Check sheet for the drawn part. Datum: minimum x, y, z corner. Units: mm. A direction names the side the tool comes from. Coordinates: 2 decimals unless noted, no trailing zeros. Write each loop counter-clockwise with the first axis right and the second up, starting at its lowest first coordinate (ties: lowest second). Pieces come first, ordered by that corner, then holes. Notation, with made-up numbers: M 78,45 L 119,45 A19 ccw 119,52 Z; hole C 34,-11.5 d4. An arc over 180 degrees is marked long. Answer in a Markdown table with one row per item.
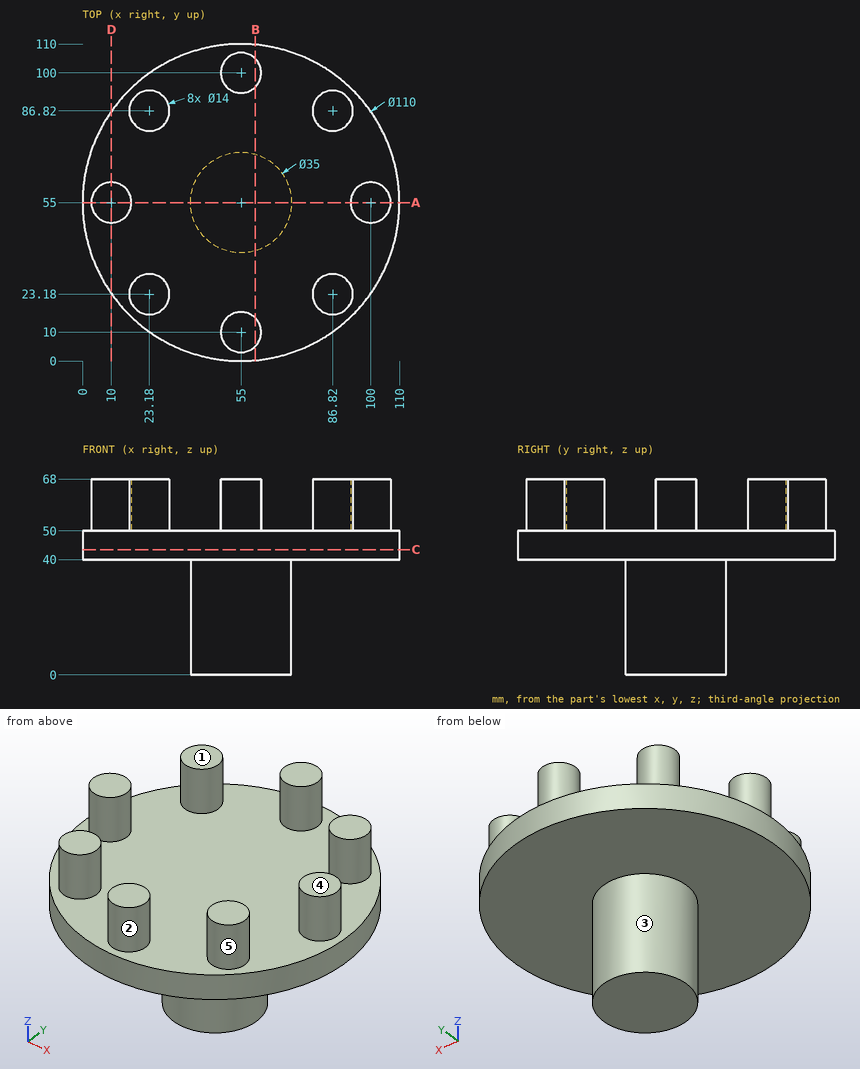
1) Sectioned sample at C-C (z = 43.5). Record the cut outline in (x, y), then the cut area to 3 significant figures.
Response values:
| item | result |
|---|---|
| outline | C 55,55 d110 |
| area | 9,500 mm² |
2) Tool access check on the marked faces 1 and 2. Record the directions out of +Z, -Z, +X, -X, +Y, -Y that give a thin tool (end or side, any length) a straight path to the whole face; none if there is none.
Response values:
| item | result |
|---|---|
| face 1 | +Z, +X, -X, +Y, -Y |
| face 2 | +Z |
3) Thickness scan on L1, parallel to Z at x = 104.5, y = 59.5; L2, parallel to Z at x = 94, y = 37; L3, parallel to Y at x = 50.5, z = 54. Record the ranges inside material, lowest first. Write a range as [from, to].
Response values:
| item | result |
|---|---|
| L1 | z = [40, 68] |
| L2 | z = [40, 50] |
| L3 | y = [4.64, 15.36], [94.64, 105.36] |
4) Sectioned sample at A-A (y = 55). Record the cut outline in (x, z).
Response values:
| item | result |
|---|---|
| outline | M 0,40 L 37.5,40 L 37.5,0 L 72.5,0 L 72.5,40 L 110,40 L 110,50 L 107,50 L 107,68 L 93,68 L 93,50 L 17,50 L 17,68 L 3,68 L 3,50 L 0,50 Z |
5) Depth check by flat-ended pin: pin 1 (10 mm diameter, centred on x = 31.5, y = 41.5, fed in from -Z); pin 2 (3 mm diameter, centred on y = 41, z = 28.5, fed in from -X); pin 3 (12 mm diameter, centred on x = 17, y = 68, fed in from +Z). Enter the tip coordinate at first touch or a pass-through.
Response values:
| item | result |
|---|---|
| pin 1 | stops at z = 40 |
| pin 2 | stops at x = 42.75 |
| pin 3 | stops at z = 50 |
6) Sectioned sample at B-B (x = 60). Record the cut outline in (y, z), then the cut area to 3 significant figures.
Response values:
| item | result |
|---|---|
| outline | M 0.23,40 L 38.23,40 L 38.23,0 L 71.77,0 L 71.77,40 L 109.77,40 L 109.77,50 L 104.9,50 L 104.9,68 L 95.1,68 L 95.1,50 L 14.9,50 L 14.9,68 L 5.1,68 L 5.1,50 L 0.23,50 Z |
| area | 2,790 mm² |
7) Release check for a two-part mould opening along X. For the marked faces 3, 4 and 5 record: +X half, -X half, draft (parallel to the pull), parting line (faces both ways), or undercut.
Response values:
| item | result |
|---|---|
| face 3 | parting line |
| face 4 | draft |
| face 5 | undercut |
8) Sectioned sample at D-D (x = 10). Record the cut outline in (y, z).
Response values:
| item | result |
|---|---|
| outline | M 23.38,40 L 86.62,40 L 86.62,50 L 62,50 L 62,68 L 48,68 L 48,50 L 23.38,50 Z |
